```python
from build123d import *

# Parameters (mm, degrees)
F1_DEPTH = 2.286
F2_R     = 0.508
F3_R     = 2.413
F4_DEPTH = 2.286


with BuildPart() as f1:
    # F0 (on Front) → F1 (new body)
    with BuildSketch(Plane.XZ):
        Polygon((39.133413, 0), (-37.066587, 0), (-37.066587, -25.4), (-11.666587, -76.2), (13.733413, -76.2), (39.133413, -25.4), align=None)
    extrude(amount=F1_DEPTH)

    # F2
    f2_edges = [f1.edges().sort_by_distance(p)[0] for p in [
        (-37.066587, -1.143, 0),
        (-37.066587, -1.143, -25.4),
        (39.133413, -1.143, 0),
        (39.133413, -1.143, -25.4),
        (13.733413, -1.143, -76.2),
        (-11.666587, -1.143, -76.2),
    ]]
    fillet(f2_edges, radius=F2_R)

    # F3 (on face) → F4 (cut)
    with BuildSketch(Plane.XZ.offset(2.286)):
        with Locations((-30.716587, -12.894039)):
            Circle(F3_R)
        with Locations((-11.666587, -12.894039)):
            Circle(F3_R)
        with Locations((13.733413, -12.894039)):
            Circle(F3_R)
        with Locations((32.783413, -12.894039)):
            Circle(F3_R)
        with Locations((1.033413, -31.75)):
            Circle(F3_R)
        with Locations((1.033413, -50.8)):
            Circle(F3_R)
        with Locations((1.033413, -69.85)):
            Circle(F3_R)
    extrude(amount=-F4_DEPTH, mode=Mode.SUBTRACT)


solid = f1.part
```
Model file for the job. Use its own axes, mm. Round coordinates to 2 decimals unless told otherwise and drop trailing zeros. Write each loop counter-clockwise with the first axis right and the second up, starting at its lowest first coordinate (ties: lowest second). Pieces come first, ordered by that corner, then holes. Notation, with made-up numbers: (87, 86.25) - (137, 86.25) arc R11 ccw to (137, 103.25) - close; hole circle Ø3 at (50, -2.75). An arc over 180 degrees is marked (long way). One line per item, written item: value.
(1) Cut at A-A, the plane z = -69.85. Give the cut face in (x, y).
Values follow:
outline: (-14.84, -2.29) - (-1.38, -2.29) - (-1.38, 0) - (-14.84, 0) - close; (3.45, -2.29) - (16.91, -2.29) - (16.91, 0) - (3.45, 0) - close
(2) Wall check: probe 1 along Z at (x, y) = (0, -1.45); probe 2 along Z at (x, y) = (-31.5, -1.8); probe 3 along Z at (x, y) = (-31, -0.7). Give the ranges that are in metal, low to high.
Values follow:
probe 1: z = -76.2 to -72.03, -67.67 to -52.98, -48.62 to -33.93, -29.57 to 0
probe 2: z = -36.53 to -15.18, -10.61 to 0
probe 3: z = -37.53 to -15.29, -10.5 to 0
(3) Two-plate mould, pull along Z, no slides. Class faces 1 (the flat face through (-24.586, -1.127, -50.36)), 2 (the flat face through (39.133, -1, -13)), 3 (the flat face through (2, -1, 0)), 4 (the cylindrical face through (0.51, -1.159, -34.106)): pulls with the +Z half, pulls with the -Z half, needs draft (parallel to the pull), parting line crosses it, or undercut.
Values follow:
face 1: pulls with the -Z half
face 2: needs draft
face 3: pulls with the +Z half
face 4: undercut
(4) Cut at B-B, the plane y = -1.45. Give the cut face in (x, z).
Values follow:
outline: (-37.07, -25.28) arc R0.51 ccw to (-37.01, -25.51) - (-11.81, -75.92) arc R0.51 ccw to (-11.35, -76.2) - (13.42, -76.2) arc R0.51 ccw to (13.87, -75.92) - (39.08, -25.51) arc R0.51 ccw to (39.13, -25.28) - (39.13, -0.51) arc R0.51 ccw to (38.63, 0) - (-36.56, 0) arc R0.51 ccw to (-37.07, -0.51) - close; hole circle Ø4.83 at (-30.72, -12.89); hole circle Ø4.83 at (-11.67, -12.89); hole circle Ø4.83 at (1.03, -69.85); hole circle Ø4.83 at (1.03, -50.8); hole circle Ø4.83 at (1.03, -31.75); hole circle Ø4.83 at (13.73, -12.89); hole circle Ø4.83 at (32.78, -12.89)
(5) Cut at C-C, the plane x = 0.5. Give the cut face in (y, z), plus the area to 3 significant figures.
Values follow:
outline: (-2.29, -76.2) - (0, -76.2) - (0, -72.2) - (-2.29, -72.2) - close; (-2.29, -67.5) - (0, -67.5) - (0, -53.15) - (-2.29, -53.15) - close; (-2.29, -48.45) - (0, -48.45) - (0, -34.1) - (-2.29, -34.1) - close; (-2.29, -29.4) - (0, -29.4) - (0, 0) - (-2.29, 0) - close
area: 142 mm²
(6) Drop a flat-ended pin along its axis: P1, Ø6.5, axis at x = 1.03, z = -69.85, coming from the +Y side. Give the stop position or say it passes through.
Values follow:
P1: stops at y = 0
(7) Cut at D-D, the plane z = -31.75. Give the cut face in (x, y).
Values follow:
outline: (-33.89, -2.29) - (-1.38, -2.29) - (-1.38, 0) - (-33.89, 0) - close; (3.45, -2.29) - (35.96, -2.29) - (35.96, 0) - (3.45, 0) - close
